Here's how the part is built. I have some questions about the finished solid (model axes, mm). Face numbers are marked on the shaded views. A direction names the side the tool comes from. Coordinates: 2 decimals unless noted, no trailing zeros. Loops run counter-clockwise (first coordinate to the right, second up) from the corner with the lowest first, then second, coordinate; pieces in that order, holes last. Notation, with made-up numbers: (51.5, 29) -> (61.5, 29) arc R21 ccw to (61.5, 52) -> close; hole circle Ø10 at (47.25, 82.5). An arc over 180 degrees is marked (long way). Answer as a JSON object with one key per item and string values. Group by question number.
Q1. I want a section at C-C on x = 21.5. Write out the boundary of the cut face in (y, z).
Q2. I want a section at A-A on y = 11.25. Write out the boundary of the cut face in (x, z), then the cut area to 3 significant figures.
Q3. Thinking about a two-plate mould opening in X: for the marked faces 4, 5 and 6, which applies, released by +X, released by -X, zero draft, split by the parting line, or undercut?
Q4. On a 3-axis mill with a long thin cutter (end or side, diameter ignored), from which of +Z, -Z, +X, -X, +Y, -Y can I reach the whole of each face in a straight line? I mean the marked faces 1, 2 and 3. Say none if no direction works.
Q5. I want a section at B-B on z = 10.5. Write out the boundary of the cut face in (x, y), then the cut area to 3 significant figures.
Q6. I'm going to push flat-ended pins straight in: pin 1 (2 mm diameter, centred on y = 17, z = 6, fed in from +X); pin 2 (4 mm diameter, centred on x = -3.5, z = 9.5, fed in from +Y). Where does each tip first touch, or does it pass through?
Q7. I need wall thicknesses on line 1 (Y direction, x = 18, z = 10.75); line 2 (X direction, y = 13.5, z = 5); line 3 (X direction, y = 18, z = 2.5). Which ranges of each line are inside material? Lowest first, please.
Q8. I want a section at D-D on y = 16.5. Write out the boundary of the cut face in (x, z).
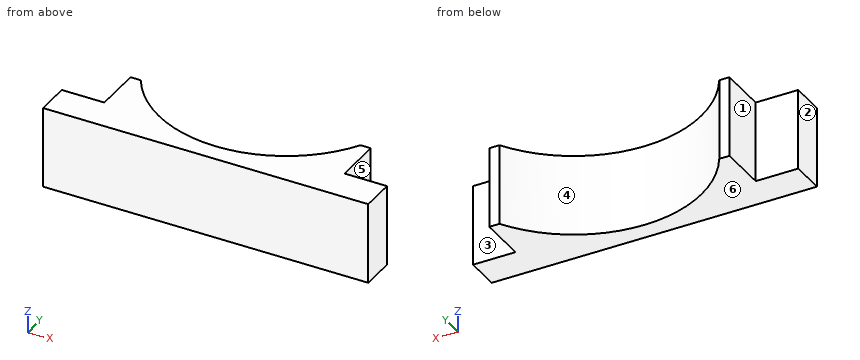
```python
from build123d import *

# Parameters (mm, degrees)
CYLINDRICAL_MOTOR_SEAT_DEPTH = 12


with BuildPart() as part:
    # Cylindrical motor seat profile → Cylindrical motor seat (new body)
    with BuildSketch(Plane.XY):
        with BuildLine():
            Line((-24, 7), (24, 7))
            Line((24, 7), (24, 12))
            Line((24, 12), (17.723131634, 12))
            Line((17.723131634, 12), (17.723131634, 19))
            Line((17.723131634, 19), (16.223131634, 19))
            ThreePointArc((16.223131634, 19), (0, 9.7), (-16.223131634, 19))
            Line((-16.223131634, 19), (-17.723131634, 19))
            Line((-17.723131634, 19), (-17.723131634, 12))
            Line((-17.723131634, 12), (-24, 12))
            Line((-24, 12), (-24, 7))
        make_face()
    extrude(amount=CYLINDRICAL_MOTOR_SEAT_DEPTH)


solid = part.part
```
Result set:
{
 "1": {"outline": "(7, 0) -> (12, 0) -> (12, 12) -> (7, 12) -> close"},
 "2": {"outline": "(-24, 0) -> (-7.48, 0) -> (-7.48, 12) -> (-24, 12) -> close; (7.48, 0) -> (24, 0) -> (24, 12) -> (7.48, 12) -> close", "area": "397 mm²"},
 "3": {"face 4": "undercut", "face 5": "released by +X", "face 6": "zero draft"},
 "4": {"face 1": "+Z, -Z, -X, +Y", "face 2": "+Z, -Z, -X, +Y, -Y", "face 3": "+Z, -Z, +X, +Y"},
 "5": {"outline": "(-24, 7) -> (24, 7) -> (24, 12) -> (17.72, 12) -> (17.72, 19) -> (16.22, 19) arc R18.8 cw to (-16.22, 19) -> (-17.72, 19) -> (-17.72, 12) -> (-24, 12) -> close", "area": "274 mm²"},
 "6": {"pin 1": "stops at x = 17.72", "pin 2": "stops at y = 10.52"},
 "7": {"line 1": "y = 7 to 12", "line 2": "x = -17.72 to -11.33, 11.33 to 17.72", "line 3": "x = -17.72 to -15.59, 15.59 to 17.72"},
 "8": {"outline": "(-17.72, 0) -> (-14.47, 0) -> (-14.47, 12) -> (-17.72, 12) -> close; (14.47, 0) -> (17.72, 0) -> (17.72, 12) -> (14.47, 12) -> close"}
}
